The model under review builds one solid part; all positions refer to its coordinate system, in mm. Face numbers are marked on the shaded views. A direction names the side the tool comes from. Coordinates: 2 decimals unless noted, no trailing zeros. Write each loop counter-clockwise with the first axis right and the second up, starting at its lowest first coordinate (ties: lowest second). Pieces come first, ordered by that corner, then holes. Notation, with made-up numbers: (-11, 26) -> (41, 26) arc R6 ccw to (41, 36) -> close; hole circle Ø2 at (-16.5, 12). An arc over 180 degrees is marked (long way). Put each result on its own line as item: value. Start each with the question number.
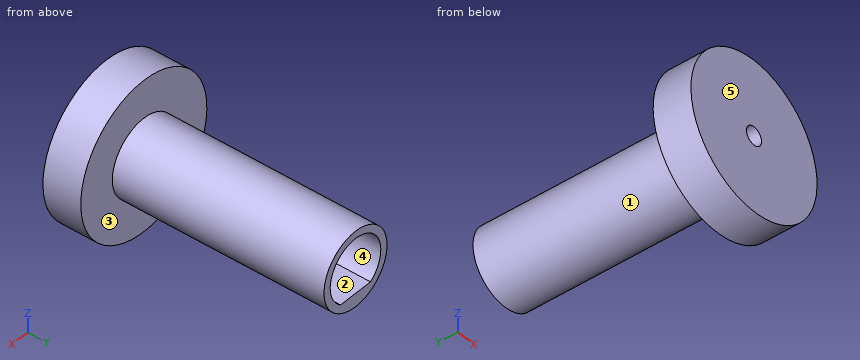
from build123d import *

# Parameters (mm, degrees)
SKETCH1_R           = 6.35
BOSS_EXTRUDE1_DEPTH = 3.175
SKETCH2_R           = 3.175
BOSS_EXTRUDE2_DEPTH = 17.78
CUT_EXTRUDE1_DEPTH  = 17.78
SKETCH4_R           = 0.762
CUT_EXTRUDE2_DEPTH  = 23.7981803


with BuildPart() as part:
    # Sketch1 → Boss-Extrude1 (new body)
    with BuildSketch(Plane(origin=(0, 0, 0), x_dir=(1, 0, 0), z_dir=(0, 1, 0))):
        with Locations(Location((0, 0, 0), (0, 0, 270))):
            Circle(SKETCH1_R)
    extrude(amount=BOSS_EXTRUDE1_DEPTH)

    # Sketch2 → Boss-Extrude2 (add)
    with BuildSketch(Plane(origin=(0, 3.175, 0), x_dir=(1, 0, 0), z_dir=(0, 1, 0))):
        with Locations(Location((0, 0, 0), (0, 0, 270))):
            Circle(SKETCH2_R)
    extrude(amount=BOSS_EXTRUDE2_DEPTH)

    # Sketch3 → Cut-Extrude1 (cut)
    with BuildSketch(Plane(origin=(0, 20.955, 0), x_dir=(1, 0, 0), z_dir=(0, 1, 0))):
        with BuildLine():
            Line((-1.516575089, 2.05), (1.516575089, 2.05))
            ThreePointArc((1.516575089, 2.05), (0, -2.55), (-1.516575089, 2.05))
        make_face()
    extrude(amount=-CUT_EXTRUDE1_DEPTH, mode=Mode.SUBTRACT)

    # Sketch4 → Cut-Extrude2 (cut, through all)
    with BuildSketch(Plane.XZ):
        with Locations(Location((0, 0, 0), (0, 0, 270))):
            Circle(SKETCH4_R)
    extrude(amount=-CUT_EXTRUDE2_DEPTH, mode=Mode.SUBTRACT)


solid = part.part
1. The part is to be moulded in two halves that separate along X. For the marked faces 1, 2 and 3, say which applies: released by +X, released by -X, zero draft, split by the parting line, or undercut.
2. Consider section D-D on z = 1.75. State the section outline as (x, y) points (3 decimals).
3. Consider section C-C on y = 12.25. State the section outline as (x, z) points (3 decimals), then the cut area to 3 significant figures.
4. Consider section A-A on z = 0. State the section outline as (x, y) points (3 decimals).
5. Insertion check: P1, Ø1.5, axis at x = 3.5, y = 16.5, coming from the +Z side; P2, Ø0.9, axis at x = 0, y = 15.5, coming from the +Z side (3 decimals); P3, Ø5, axis at x = 1.5, y = 16, coming from the -Z side (3 decimals). Each pin has a flat end and moves straight along its axis. Give the tip position at first contact, or say it passes through.
6. Consider section B-B on x = 0. State the section outline as (y, z) points (3 decimals), then the cut area to 3 significant figures.
7. Wall thickness on line 1 (X direction, y = 1.3, z = 0); line 2 (X direction, y = 16, z = 0) (3 decimals); line 3 (Y direction, x = 4, z = -0.25) (3 decimals): over which ranges is each line inside the solid? List them lowest first. Write a range as from..to.
8. Tool access review of the marked faces 4 and 5: name each direction out of +Z, -Z, +X, -X, +Y, -Y from which nothing blocks a thin tool from reaching the whole face with its end or side.
Output values:
1. face 1: split by the parting line
1. face 2: undercut
1. face 3: zero draft
2. outline: (-6.104, 0) -> (6.104, 0) -> (6.104, 3.175) -> (2.649, 3.175) -> (2.649, 20.955) -> (1.855, 20.955) -> (1.855, 3.175) -> (-1.855, 3.175) -> (-1.855, 20.955) -> (-2.649, 20.955) -> (-2.649, 3.175) -> (-6.104, 3.175) -> close
3. outline: circle Ø6.35 at (0, 0); hole (-1.517, -2.05) -> (1.517, -2.05) arc R2.55 ccw (long way) to start
3. area: 12.3 mm^2
4. outline: (-6.35, 0) -> (-0.762, 0) -> (-0.762, 3.175) -> (-2.55, 3.175) -> (-2.55, 20.955) -> (-3.175, 20.955) -> (-3.175, 3.175) -> (-6.35, 3.175) -> close; (0.762, 0) -> (6.35, 0) -> (6.35, 3.175) -> (3.175, 3.175) -> (3.175, 20.955) -> (2.55, 20.955) -> (2.55, 3.175) -> (0.762, 3.175) -> close
5. P1: stops at z = 1.59
5. P2: stops at z = 3.175
5. P3: stops at z = -3.175
6. outline: (0, -6.35) -> (3.175, -6.35) -> (3.175, -3.175) -> (20.955, -3.175) -> (20.955, -2.05) -> (3.175, -2.05) -> (3.175, -0.762) -> (0, -0.762) -> close; (0, 0.762) -> (3.175, 0.762) -> (3.175, 2.55) -> (20.955, 2.55) -> (20.955, 3.175) -> (3.175, 3.175) -> (3.175, 6.35) -> (0, 6.35) -> close
6. area: 66.6 mm^2
7. line 1: x = -6.35..-0.76, 0.76..6.35
7. line 2: x = -3.175..-2.55, 2.55..3.175
7. line 3: y = 0..3.175
8. face 4: +Y
8. face 5: +Z, -Z, +X, -X, -Y
